```python
from build123d import *

# Parameters (mm, degrees)
F0_R     = 8
F1_DEPTH = 15
F3_DEPTH = 12.5
F4_DEPTH = 5


with BuildPart() as f1:
    # F0 (on Top) → F1 (new body)
    with BuildSketch(Plane.XY):
        Circle(F0_R)
        with BuildLine():
            ThreePointArc((0.3998477713, 7.2389655172), (5.1265241636, 5.1265241636), (7.2389655172, 0.3998477713))
            ThreePointArc((7.2389655172, 0.3998477713), (7.5289141507, 0.2867174507), (7.65, 0))
            ThreePointArc((7.65, 0), (7.5289141507, -0.2867174507), (7.2389655172, -0.3998477713))
            ThreePointArc((7.2389655172, -0.3998477713), (5.1265241636, -5.1265241636), (0.3998477713, -7.2389655172))
            ThreePointArc((0.3998477713, -7.2389655172), (0.399961941, -7.2444822336), (0.4, -7.25))
            ThreePointArc((0.4, -7.25), (-0.0055177664, -7.649961941), (-0.3998477713, -7.2389655172))
            ThreePointArc((-0.3998477713, -7.2389655172), (-5.1265241636, -5.1265241636), (-7.2389655172, -0.3998477713))
            ThreePointArc((-7.2389655172, -0.3998477713), (-7.65, 0), (-7.2389655172, 0.3998477713))
            ThreePointArc((-7.2389655172, 0.3998477713), (-5.1265241636, 5.1265241636), (-0.3998477713, 7.2389655172))
            ThreePointArc((-0.3998477713, 7.2389655172), (-0.0055177664, 7.649961941), (0.4, 7.25))
            ThreePointArc((0.4, 7.25), (0.399961941, 7.2444822336), (0.3998477713, 7.2389655172))
        make_face(mode=Mode.SUBTRACT)
        with BuildLine():
            ThreePointArc((-7.2389655172, -0.3998477713), (-7.25, 0), (-7.2389655172, 0.3998477713))
            ThreePointArc((-7.2389655172, 0.3998477713), (-7.65, 0), (-7.2389655172, -0.3998477713))
        make_face()
        with BuildLine():
            ThreePointArc((0.4, -7.25), (0.399961941, -7.2444822336), (0.3998477713, -7.2389655172))
            ThreePointArc((0.3998477713, -7.2389655172), (0, -7.25), (-0.3998477713, -7.2389655172))
            ThreePointArc((-0.3998477713, -7.2389655172), (-0.0055177664, -7.649961941), (0.4, -7.25))
        make_face()
        with BuildLine():
            ThreePointArc((7.2389655172, 0.3998477713), (7.2472408543, 0.2), (7.25, 0))
            ThreePointArc((7.25, 0), (7.2472408543, -0.2), (7.2389655172, -0.3998477713))
            ThreePointArc((7.2389655172, -0.3998477713), (7.5289141507, -0.2867174507), (7.65, 0))
            ThreePointArc((7.65, 0), (7.5289141507, 0.2867174507), (7.2389655172, 0.3998477713))
        make_face()
        with BuildLine():
            ThreePointArc((-0.3998477713, 7.2389655172), (0, 7.25), (0.3998477713, 7.2389655172))
            ThreePointArc((0.3998477713, 7.2389655172), (0.399961941, 7.2444822336), (0.4, 7.25))
            ThreePointArc((0.4, 7.25), (-0.0055177664, 7.649961941), (-0.3998477713, 7.2389655172))
        make_face()
    extrude(amount=F1_DEPTH)

    # F2 (on Right) → F3 (cut, symmetric)
    with BuildSketch(Plane.YZ):
        Polygon((-8, 15), (-8, 5), (8, 15), align=None)
        with BuildLine():
            Line((8, 15), (-8, 5))
            ThreePointArc((-8, 5), (1.6308873071, 7.3905803087), (8, 15))
        make_face()
    extrude(amount=F3_DEPTH, both=True, mode=Mode.SUBTRACT)

    # F0 (on Top) → F4 (join)
    with BuildSketch(Plane.XY):
        with BuildLine():
            ThreePointArc((-6.85, 0), (-6.9632825493, 0.2789141507), (-7.2389655172, 0.3998477713))
            ThreePointArc((-7.2389655172, 0.3998477713), (-7.25, 0), (-7.2389655172, -0.3998477713))
            ThreePointArc((-7.2389655172, -0.3998477713), (-6.9632825493, -0.2789141507), (-6.85, 0))
        make_face()
        with BuildLine():
            ThreePointArc((-0.3998477713, -7.2389655172), (0, -7.25), (0.3998477713, -7.2389655172))
            ThreePointArc((0.3998477713, -7.2389655172), (0, -6.85), (-0.3998477713, -7.2389655172))
        make_face()
        with BuildLine():
            ThreePointArc((7.2389655172, -0.3998477713), (7.2472408543, -0.2), (7.25, 0))
            ThreePointArc((7.25, 0), (7.2472408543, 0.2), (7.2389655172, 0.3998477713))
            ThreePointArc((7.2389655172, 0.3998477713), (6.85, 0), (7.2389655172, -0.3998477713))
        make_face()
        with BuildLine():
            ThreePointArc((-0.3998477713, 7.2389655172), (0, 6.85), (0.3998477713, 7.2389655172))
            ThreePointArc((0.3998477713, 7.2389655172), (0, 7.25), (-0.3998477713, 7.2389655172))
        make_face()
    extrude(amount=F4_DEPTH)


solid = f1.part
```
Build history of the part. All positions in model axes, mm. Coordinates: 2 decimals unless noted, no trailing zeros. Order: outer loops, then holes, each group sorted by start corner. A loop starts at its lowest first (then second) coordinate and runs counter-clockwise, first axis right, second up.
Item 1: Drill centre lines: L1, parallel to Z at x = 3.25, y = -7; L2, parallel to X at y = 6.5, z = 6.75; L3, parallel to X at y = -4.75, z = 3.25. Where is each one in solid material? Low to high.
Filled in:
L1: z = 0 to 4.96
L2: x = -4.66 to -3.21, 3.21 to 4.66
L3: x = -6.44 to -5.48, 5.48 to 6.44
Item 2: Saw through at D-D on y = 5.75. List the corners of the cut face in (x, z).
Filled in:
outline: (-5.56, 0) - (-4.42, 0) - (-4.42, 11.1) - (-5.56, 11.1) - close; (4.42, 0) - (5.56, 0) - (5.56, 11.1) - (4.42, 11.1) - close
Item 3: Saw through at C-C on z = 3.5. List the corners of the cut face in (x, y).
Filled in:
outline: circle Ø16 at (0, 0); hole (-7.24, -0.4) arc R7.25 ccw to (-0.4, -7.24) arc R0.4 cw to (0.4, -7.24) arc R7.25 ccw to (7.24, -0.4) arc R0.4 cw to (7.24, 0.4) arc R7.25 ccw to (0.4, 7.24) arc R0.4 cw to (-0.4, 7.24) arc R7.25 ccw to (-7.24, 0.4) arc R0.4 cw to start
Item 4: Drop flat-ended pins along their axis: pin 1 Ø6 at (x, z) = (2.5, 9) entering from -Y; pin 2 Ø1.5 at (x, z) = (4, 3) entering from -Y; pin 3 Ø6 at (y, z) = (2.5, 9.5) entering from +X. Give the stop position or say it passes through.
Filled in:
pin 1: stops at y = 4.72
pin 2: stops at y = -7.31
pin 3: stops at x = 7.95
Item 5: Saw through at A-A on y = 1.5. List the corners of the cut face in (x, z), then the cut area to 3 significant figures.
Filled in:
outline: (-7.86, 0) - (-7.09, 0) - (-7.09, 7.31) - (-7.86, 7.31) - close; (7.09, 0) - (7.86, 0) - (7.86, 7.31) - (7.09, 7.31) - close
area: 11.2 mm2
